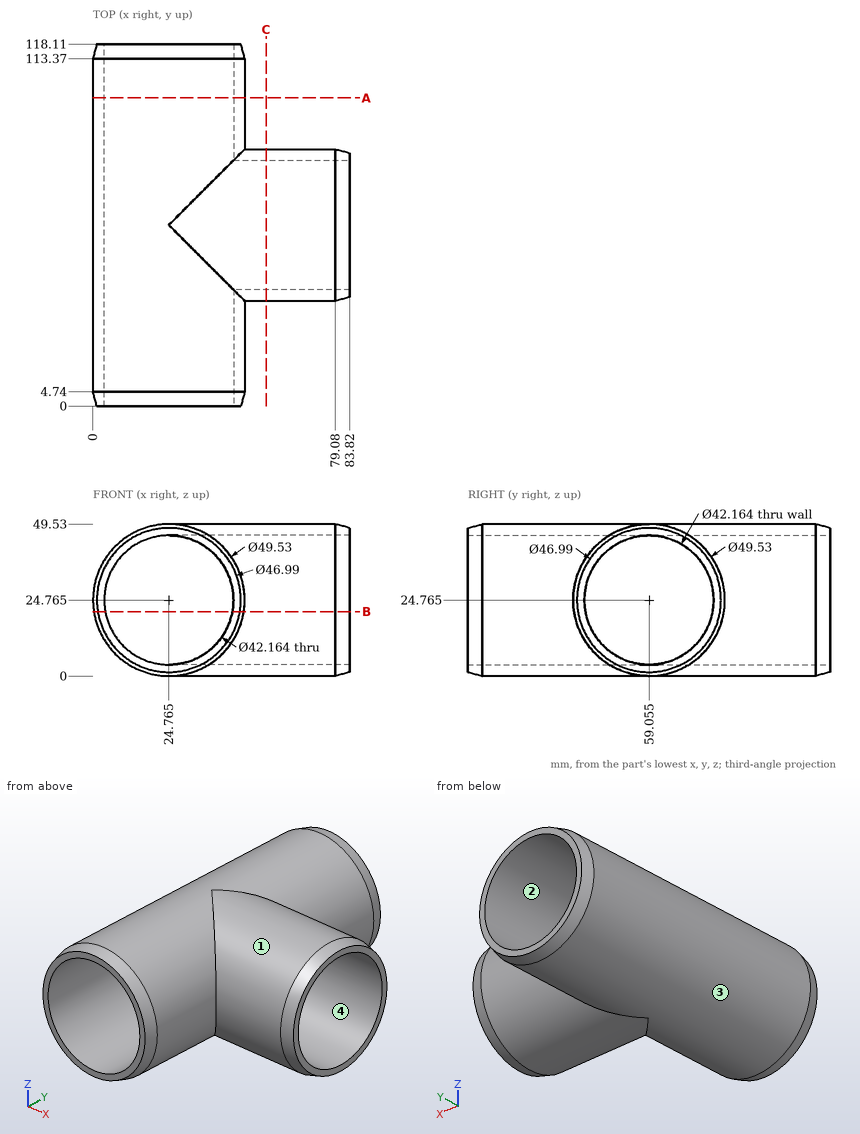
Geometry: see drawing. Coordinates: mm, zero at the bounding-box minimum. A direction names the side the tool comes from. Coordinates: 2 decimals unless noted, no trailing zeros. Write each loop counter-clockwise with the first axis right and the second up, starting at its lowest first coordinate (ties: lowest second). Pieces come first, ordered by that corner, then holes.
1) Mould query, pull axis Z, two halves, no side actions, for the marked faces 3 and 4. Classes: pulls with the +Z half, pulls with the -Z half, needs draft (parallel to the pull), parting line crosses it, or undercut.
2) Pin query (flat end, axial travel): pin 1 Ø1.5 at (y, z) = (65.5, 23) entering from -X; pin 2 Ø5 at (y, z) = (72, 17) entering from +X; pin 3 Ø12 at (x, z) = (64, 18) entering from +Y. Return the tip coordinate at first contact, or that it passes through.
3) Section A-A on y = 100.5. Output: boundary loops of the cut face in (x, z) (1 decimal).
4) Material intervals for line 1 along X through (y, z) = (98.5, 24); line 2 along Z through (x, y) = (25, 16.5); line 3 along Y through (x, z) = (73, 32), sorted ascending.
5) Set-up query: the marked faces 1 and 2. Return all of +Z, -Z, +X, -X, +Y, -Y with unobstructed straight access to the full face (end or side cutting, diameter ignored); none if empty.
6) Section B-B on z = 21. State how many separate pieces and enclosed holes the cut face has, and give its area (3 significant figures).
7) Section C-C on x = 56.5. Output: boundary loops of the cut face in (y, z) (1 decimal).
Check result:
1. face 3: parting line crosses it
1. face 4: undercut
2. pin 1: stops at x = 0.02
2. pin 2: stops at x = 6.35
2. pin 3: stops at y = 83.81
3. outline: circle Ø49.5 at (24.8, 24.8); hole circle Ø42.2 at (24.8, 24.8)
4. line 1: x = 0.01 to 3.7, 45.83 to 49.52
4. line 2: z = 0 to 3.68, 45.85 to 49.53
4. line 3: y = 35.37 to 39.25, 78.86 to 82.74
5. face 1: +X
5. face 2: +Y, -Y
6. separate pieces: 3
6. enclosed holes: 0
6. area: 967 mm2
7. outline: circle Ø49.5 at (59.1, 24.8); hole circle Ø42.2 at (59.1, 24.8)
